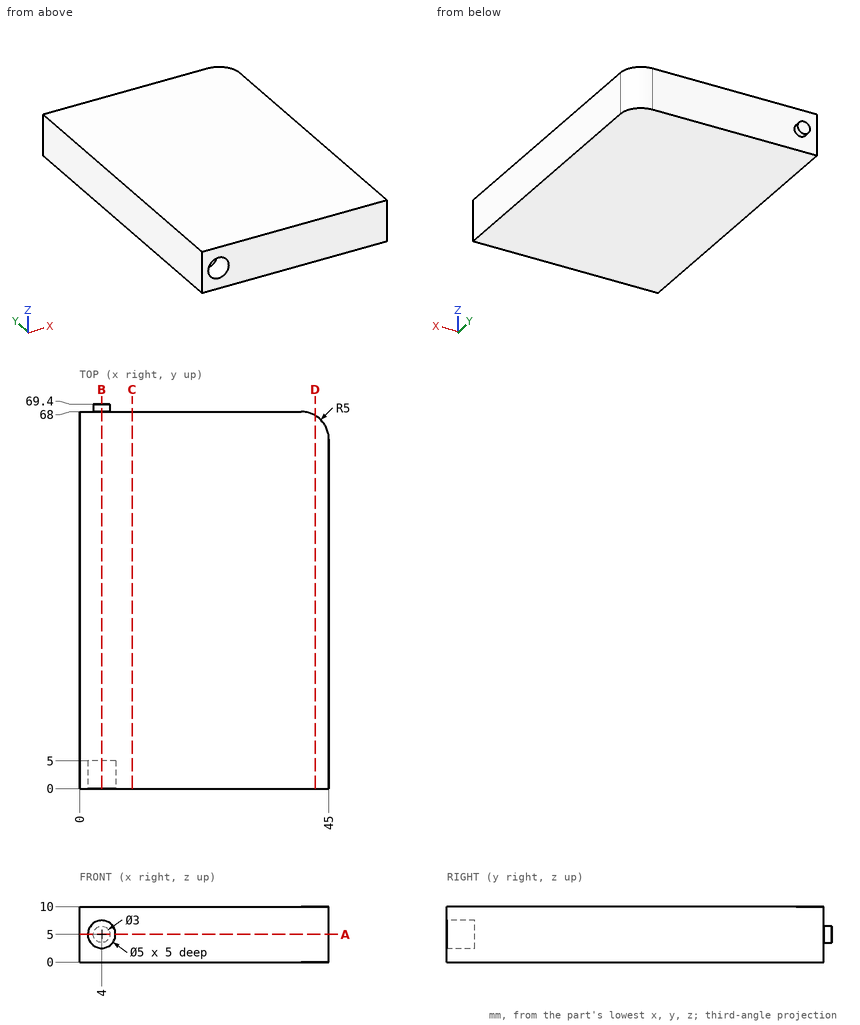
For this review, use the dimensioned drawing (mm, ordinates from the lowest corner) and the shaded views. Give positions to 0.01 mm unless a question says otherwise; leave off trailing zeros. Loops run counter-clockwise (first coordinate to the right, second up) from the corner with the lowest first, then second, coordinate; pieces in that order, holes last.
Item 1: For line 1 along Y through (x, z) = (38, 4.25); line 2 along Y through (x, z) = (2, 5.5), list the stretches that pass through material, from the lowest coordinate up.
Item 2: Take a section at B-B, the plane x = 4. State the section outline as (y, z) points, and give its area (3 significant figures).
Item 3: Insertion check: pin 1 (8 mm diameter, centred on x = 8, y = 44.5, fed in from -Z). The pin has a flat end and moves straight along its axis. Give the tip position at first contact, or say it passes through.
Item 4: Take a section at A-A, the plane z = 5. State the section outline as (x, y) points.
Item 5: Take a section at D-D, the plane x = 42.5. State the section outline as (y, z) points.
Item 6: Take a section at C-C, the plane x = 9.5. State the section outline as (y, z) points, and give its area (3 significant figures).
Calculated:
1. line 1: y = 0 to 68
1. line 2: y = 5 to 68
2. outline: (0, 0) - (68, 0) - (68, 3.5) - (69.4, 3.5) - (69.4, 6.5) - (68, 6.5) - (68, 10) - (0, 10) - (0, 7.5) - (5, 7.5) - (5, 2.5) - (0, 2.5) - close
2. area: 659 mm2
3. pin 1: stops at z = 0
4. outline: (0, 0) - (1.5, 0) - (1.5, 5) - (6.5, 5) - (6.5, 0) - (45, 0) - (45, 63) arc R5 ccw to (40, 68) - (5.5, 68) - (5.5, 69.4) - (2.5, 69.4) - (2.5, 68) - (0, 68) - close
5. outline: (0, 0) - (67.33, 0) - (67.33, 10) - (0, 10) - close
6. outline: (0, 0) - (68, 0) - (68, 10) - (0, 10) - close
6. area: 680 mm2
